from build123d import *

# Parameters (mm, degrees)
SKETCH1_W           = 108.5
SKETCH1_H           = 29.5
BOSS_EXTRUDE1_DEPTH = 2
SKETCH2_R           = 1.75
CUT_EXTRUDE1_DEPTH  = 3
FILLET1_R           = 3
SKETCH5_R           = 2
SKETCH5_W           = 16
SKETCH5_H           = 14
SKETCH5_W_2         = 15.2
SKETCH5_H_2         = 7.6
SKETCH5_W_3         = 1.1
SKETCH5_H_3         = 0.4
SKETCH5_W_4         = 9
SKETCH5_H_4         = 11.5
CUT_EXTRUDE2_DEPTH  = 3
FILLET2_R           = 1
FILLET3_R           = 1.5
FILLET4_R           = 0.5


with BuildPart() as part:
    # Sketch1 → Boss-Extrude1 (new body)
    with BuildSketch(Plane(origin=(0, 0, 0), x_dir=(1, 0, 0), z_dir=(0, 1, 0))):
        with Locations((54.25, 14.75)):
            Rectangle(SKETCH1_W, SKETCH1_H)
    extrude(amount=BOSS_EXTRUDE1_DEPTH)

    # Sketch2 → Cut-Extrude1 (cut, through all)
    with BuildSketch(Plane(origin=(0, 2, 0), x_dir=(1, 0, 0), z_dir=(0, 1, 0))):
        with Locations((6, 26.45)):
            Circle(SKETCH2_R)
        with Locations((6, 4.95)):
            Circle(SKETCH2_R)
        with Locations((102.5, 4.95)):
            Circle(SKETCH2_R)
        with Locations((102.5, 26.45)):
            Circle(SKETCH2_R)
    extrude(amount=-CUT_EXTRUDE1_DEPTH, mode=Mode.SUBTRACT)

    # Fillet1
    fillet1_edges = [part.edges().sort_by_distance(p)[0] for p in [
        (0, 1, -29.5),
        (108.5, 1, -29.5),
        (108.5, 1, 0),
        (0, 1, 0),
    ]]
    fillet(fillet1_edges, radius=FILLET1_R)

    # Sketch5 → Cut-Extrude2 (cut, through all)
    with BuildSketch(Plane(origin=(0, 2, 0), x_dir=(1, 0, 0), z_dir=(0, 1, 0))):
        with Locations((94.303253972, 15)):
            Circle(SKETCH5_R)
        with Locations((21.75, 11.2)):
            Rectangle(SKETCH5_W, SKETCH5_H)
        with Locations((43.2, 14)):
            Rectangle(SKETCH5_W_2, SKETCH5_H_2)
        Polygon((55.903253972, 18.2), (55.903253972, 15.2), (64.403253972, 15.2), (64.403253972, 18.2), (64.403253972, 18.7), (55.903253972, 18.7), align=None)
        with Locations((89.453253972, 18)):
            Rectangle(SKETCH5_W_3, SKETCH5_H_3)
        Polygon((67.903253972, 18.2), (67.903253972, 15.2), (76.403253972, 15.2), (76.403253972, 18.2), (76.403253972, 18.7), (67.903253972, 18.7), align=None)
        with Locations((82.903253972, 12.45)):
            Rectangle(SKETCH5_W_4, SKETCH5_H_4)
    extrude(amount=-CUT_EXTRUDE2_DEPTH, mode=Mode.SUBTRACT)

    # Fillet2
    fillet2_edges = [part.edges().sort_by_distance(p)[0] for p in [
        (50.8, 1, -10.2),
        (35.6, 1, -10.2),
        (35.6, 1, -17.8),
        (50.8, 1, -17.8),
    ]]
    fillet(fillet2_edges, radius=FILLET2_R)

    # Fillet3
    fillet3_edges = [part.edges().sort_by_distance(p)[0] for p in [
        (67.903253972, 1, -18.7),
        (76.403253972, 1, -18.7),
        (55.903253972, 1, -18.7),
        (64.403253972, 1, -18.7),
    ]]
    fillet(fillet3_edges, radius=FILLET3_R)

    # Fillet4
    fillet4_edges = [part.edges().sort_by_distance(p)[0] for p in [
        (76.403253972, 1, -15.2),
        (67.903253972, 1, -15.2),
        (64.403253972, 1, -15.2),
        (55.903253972, 1, -15.2),
    ]]
    fillet(fillet4_edges, radius=FILLET4_R)


solid = part.part
Read the model definition and answer for the solid it produces. Units are mm, in the model's axes. A direction names the side the tool comes from. Coordinates: 2 decimals unless noted, no trailing zeros. Write each loop counter-clockwise with the first axis right and the second up, starting at its lowest first coordinate (ties: lowest second). Pieces come first, ordered by that corner, then holes. Notation, with made-up numbers: M 63.25,83 L 88.25,83 A25 cw 88.25,116 Z; hole C -18.75,-35.5 d11. An arc over 180 degrees is marked long. Use a Markdown table: item, result.
Q1. The part is cut by section C-C, the plane x = 21.5. Write down the section's boundary in (y, z).
Answer block:
| item | result |
|---|---|
| outline | M 0,-29.5 L 2,-29.5 L 2,-18.2 L 0,-18.2 Z; M 0,-4.2 L 2,-4.2 L 2,0 L 0,0 Z |
Q2. This flat-tipped pin is pushed along its axis until it touches: pin 1 Ø3 at (x, z) = (102.5, -26.45) entering from -Y. Where does it stop, or does it pass through?
Answer block:
| item | result |
|---|---|
| pin 1 | passes through |
Q3. The part is cut by section A-A, the plane x = 85. Write down the section's boundary in (y, z).
Answer block:
| item | result |
|---|---|
| outline | M 0,-29.5 L 2,-29.5 L 2,-18.2 L 0,-18.2 Z; M 0,-6.7 L 2,-6.7 L 2,0 L 0,0 Z |
Q4. The part is cut by section D-D, the plane y = 0.65. Give the number of separate pieces and of enclosed holes in the cut face, then the cut area to 3 significant figures.
Answer block:
| item | result |
|---|---|
| separate pieces | 1 |
| enclosed holes | 11 |
| area | 2,640 mm2 |
Q5. Straight lines are drawn through the part: L1, parallel to X at y = 1.35, z = -26.45; L2, parallel to X at y = 1.65, z = -4.75; L3, parallel to Z at x = 6, y = 1.1. For each, find the intervals that lie inside material, in ascending order. Write a range as [from, to].
Answer block:
| item | result |
|---|---|
| L1 | x = [0, 4.25], [7.75, 100.75], [104.25, 108.5] |
| L2 | x = [0, 4.26], [7.74, 13.75], [29.75, 100.76], [104.24, 108.5] |
| L3 | z = [-29.5, -28.2], [-24.7, -6.7], [-3.2, 0] |
Q6. Determine the mould class of faces 1 (the face through (13.75, 1, -11)), 2 (the face through (108.5, 1, -15)), 3 (the face through (54, 1, -29.5)) for opening direction X: released by +X, released by -X, zero draft, split by the parting line, or undercut.
Answer block:
| item | result |
|---|---|
| face 1 | undercut |
| face 2 | released by +X |
| face 3 | zero draft |
Q7. The part is cut by section B-B, the plane x = 102.5. Write down the section's boundary in (y, z).
Answer block:
| item | result |
|---|---|
| outline | M 0,-29.5 L 2,-29.5 L 2,-28.2 L 0,-28.2 Z; M 0,-24.7 L 2,-24.7 L 2,-6.7 L 0,-6.7 Z; M 0,-3.2 L 2,-3.2 L 2,0 L 0,0 Z |
Q8. Which of the six approach directions +Z, -Z, +X, -X, +Y, -Y give full straight-line access (tool end or side, diameter ignored) to faces 4 (the face through (53, 2, -15)), 5 (the face through (60, 1, -18.7))?
Answer block:
| item | result |
|---|---|
| face 4 | +Z, -Z, +X, -X, +Y |
| face 5 | +Y, -Y |
